from build123d import *

# Parameters (mm, degrees)
SKETCH1_R           = 4
BOSS_EXTRUDE1_DEPTH = 2.54
SKETCH2_R           = 1.09
CUT_EXTRUDE1_DEPTH  = 5
CIRPATTERN1_COUNT   = 8
SKETCH3_R           = 1.27
BOSS_EXTRUDE2_DEPTH = 2.54
FILLET1_R           = 1


with BuildPart() as part:
    # Sketch1 → Boss-Extrude1 (new body)
    with BuildSketch(Plane(origin=(0, 0, 0), x_dir=(1, 0, 0), z_dir=(0, 1, 0))):
        with BuildLine():
            Line((-19.24, 0), (-19.24, -25.4))
            Line((-19.24, -25.4), (19.24, -25.4))
            Line((19.24, -25.4), (19.24, 0))
            ThreePointArc((19.24, 0), (0, 19.24), (-19.24, 0))
        make_face()
        with Locations(Location((0, 0, 0), (0, 0, 270))):
            Circle(SKETCH1_R, mode=Mode.SUBTRACT)
    extrude(amount=BOSS_EXTRUDE1_DEPTH)

    # Sketch2 → Cut-Extrude1 (cut, symmetric)
    with BuildSketch(Plane(origin=(0, 2.54, 0), x_dir=(1, 0, 0), z_dir=(0, 1, 0))):
        with Locations(Location((0, 8.5, 0), (0, 0, 270))):
            Circle(SKETCH2_R)
    cut_extrude1 = extrude(amount=CUT_EXTRUDE1_DEPTH, both=True, mode=Mode.SUBTRACT)

    # CirPattern1: Cut-Extrude1 ×8 about axis
    cirpattern1_axis = Axis((0, 0, 0), (0, 1, 0))
    for i in range(1, CIRPATTERN1_COUNT):
        add(cut_extrude1.rotate(cirpattern1_axis, i * 360 / CIRPATTERN1_COUNT), mode=Mode.SUBTRACT)

    # Sketch3 → Boss-Extrude2 (add)
    with BuildSketch(Plane.XY.offset(25.4)):
        with BuildLine():
            Line((19.24, 2.54), (19.24, 25.4))
            ThreePointArc((19.24, 25.4), (0, 44.64), (-19.24, 25.4))
            Line((-19.24, 25.4), (-19.24, 2.54))
            Line((-19.24, 2.54), (19.24, 2.54))
        make_face()
        with Locations((6.35, 37.62)):
            Circle(SKETCH3_R, mode=Mode.SUBTRACT)
        with Locations((6.35, 11.62)):
            Circle(SKETCH3_R, mode=Mode.SUBTRACT)
        with Locations(Location((-6.35, 11.62, 0), (0, 0, 180))):
            Circle(SKETCH3_R, mode=Mode.SUBTRACT)
        with Locations(Location((-6.35, 37.62, 0), (0, 0, 180))):
            Circle(SKETCH3_R, mode=Mode.SUBTRACT)
        with BuildLine():
            Line((6.35, 32.24), (6.35, 17))
            ThreePointArc((6.35, 17), (0, 10.65), (-6.35, 17))
            Line((-6.35, 17), (-6.35, 32.24))
            ThreePointArc((-6.35, 32.24), (0, 38.59), (6.35, 32.24))
        make_face(mode=Mode.SUBTRACT)
        with BuildLine():
            Line((14.66, 25.89), (12.12, 25.89))
            ThreePointArc((12.12, 25.89), (10.85, 24.62), (12.12, 23.35))
            Line((12.12, 23.35), (14.66, 23.35))
            ThreePointArc((14.66, 23.35), (15.93, 24.62), (14.66, 25.89))
        make_face(mode=Mode.SUBTRACT)
        with BuildLine():
            Line((-14.66, 23.35), (-12.12, 23.35))
            ThreePointArc((-12.12, 23.35), (-10.85, 24.62), (-12.12, 25.89))
            Line((-12.12, 25.89), (-14.66, 25.89))
            ThreePointArc((-14.66, 25.89), (-15.93, 24.62), (-14.66, 23.35))
        make_face(mode=Mode.SUBTRACT)
    extrude(amount=-BOSS_EXTRUDE2_DEPTH)

    # Fillet1
    fillet1_edges = [part.edges().sort_by_distance(p)[0] for p in [
        (0, 0, 25.4),
        (0, 2.54, 22.86),
    ]]
    fillet(fillet1_edges, radius=FILLET1_R)


solid = part.part
The listing builds one solid part. Answer for the finished solid, in the listing's coordinates (mm). A direction names the side the tool comes from. Round coordinates to 2 decimals unless told otherwise and drop trailing zeros. Order: outer loops, then holes, each group sorted by start corner. A loop starts at its lowest first (then second) coordinate and runs counter-clockwise, first axis right, second up. Notation, with made-up numbers: (57.5, 65.25) - (86.5, 65.25) arc R18 cw to (86.5, 95.25) - close; hole circle Ø11 at (81, -33.5). An arc over 180 degrees is marked (long way). Write item = value, one per line. Start each with the question number.
1) Section C-C, the plane x = 0 is taken. Write down the section's boundary in (y, z), plus the area to 3 significant figures.
2) Straight lines are drawn through the part: L1, parallel to Y at x = -10.5, z = -16; L2, parallel to Z at x = 1, y = 8.5; L3, parallel to Z at x = 8.5, y = 1. For each, find the intervals that lie inside material, in ascending order.
3) Given pin 1 (3 mm diameter, centred on x = 13, z = 24, fed in from +Y); pin 2 (3.5 mm diameter, centred on x = 6.35, y = 11.62, fed in from -Z); pin 3 (1 mm diameter, centred on x = -12.5, z = -7.5, fed in from +Y); pin 4 (3 mm diameter, centred on x = 6.01, z = -6.01, fed in from -Y), each flat-ended and moving along its own axis, determine where each tip first touches the part or whether it passes through.
4) Section B-B, the plane y = 19 is taken. Write down the section's boundary in (x, z), plus the area to 3 significant figures.
5) Section A-A, the plane z = 8.5 is taken. Write down the section's boundary in (x, y), plus the area to 3 significant figures.
6) For a pull along Y with two mould halves and no side action, classify faces 1 (the flat face through (0, 2.54, 6)), 2 (the cylindrical face through (4.97, 1.29, -6.34)), 3 (the cylindrical face through (-0.14, 38.59, 24.15)), 4 (the cylindrical face through (10.85, 24.65, 24.15)) as released by +Y, released by -Y, zero draft, split by the parting line, or undercut.
7) Section D-D, the plane y = 11.62 is taken. Write down the section's boundary in (x, z).
8) For faces 5 (the flat face through (13, 25.89, 24)), 6 (the cylindrical face through (-6.34, 1.29, -4.97)), determine the directions among +Z, -Z, +X, -X, +Y, -Y from which every point of the face is accessible in a straight line to the end or side of a thin tool.
Results list:
q1.outline = (0, -19.24) - (2.54, -19.24) - (2.54, -9.59) - (0, -9.59) - close; (0, -7.41) - (2.54, -7.41) - (2.54, -4) - (0, -4) - close; (0, 4) - (2.54, 4) - (2.54, 7.41) - (0, 7.41) - close; (0, 9.59) - (2.54, 9.59) - (2.54, 21.86) arc R1 cw to (3.54, 22.86) - (10.65, 22.86) - (10.65, 25.4) - (1, 25.4) arc R1 ccw to (0, 24.4) - close; (38.59, 22.86) - (44.64, 22.86) - (44.64, 25.4) - (38.59, 25.4) - close
q1.area = 118 mm^2
q2.L1 = 0 to 2.54
q2.L2 = 22.86 to 25.4
q2.L3 = -17.26 to -1.09, 1.09 to 25.4
q3.pin_1 = 40.82
q3.pin_2 = 22.86
q3.pin_3 = 2.54
q3.pin_4 = 0
q4.outline = (-19.24, 22.86) - (-6.35, 22.86) - (-6.35, 25.4) - (-19.24, 25.4) - close; (6.35, 22.86) - (19.24, 22.86) - (19.24, 25.4) - (6.35, 25.4) - close
q4.area = 65.5 mm^2
q5.outline = (-19.24, 0) - (-1.09, 0) - (-1.09, 2.54) - (-19.24, 2.54) - close; (1.09, 0) - (19.24, 0) - (19.24, 2.54) - (1.09, 2.54) - close
q5.area = 92.2 mm^2
q6.face_1 = released by +Y
q6.face_2 = zero draft
q6.face_3 = undercut
q6.face_4 = undercut
q7.outline = (-19.24, 22.86) - (-7.62, 22.86) - (-7.62, 25.4) - (-19.24, 25.4) - close; (-5.08, 22.86) - (-3.37, 22.86) - (-3.37, 25.4) - (-5.08, 25.4) - close; (3.37, 22.86) - (5.08, 22.86) - (5.08, 25.4) - (3.37, 25.4) - close; (7.62, 22.86) - (19.24, 22.86) - (19.24, 25.4) - (7.62, 25.4) - close
q8.face_5 = +Z, -Z
q8.face_6 = +Y, -Y
